Verification items for the finished model (mm, model axes). Coordinates: 2 decimals unless noted, no trailing zeros. Order: outer loops, then holes, each group sorted by start corner. A loop starts at its lowest first (then second) coordinate and runs counter-clockwise, first axis right, second up. Notation, with made-up numbers: (-40, 40) -> (-11, 40) arc R10 cw to (-11, 47) -> close; hole circle Ø4 at (39.25, 49). An arc over 180 degrees is marked (long way). Write each question's results on one line, items separated by ' | '. Start each with the question number.
(1) Cross-section at D-D on x = -12.5. Enter the section's corners in (y, z).
(2) Draft check along X on faces 1 (the cylindrical face through (-5.69, 9.84, 78.54)), 2 (the flat face through (-9, 44, 81)), 3 (the flat face through (-71.5, 46, 78)). Enter one of: +X half, -X half, draft (parallel to the pull), parting line (faces both ways), or undercut.
(3) Thickness scan on probe 1 along Y at (x, z) = (-37.5, 79.15); probe 2 along Y at (x, z) = (-12.5, 78.4); probe 3 along X at (y, z) = (70, 78.9). Record the ranges inside material, lowest first. Write a range as [from, to].
(4) Cross-section at B-B on y = 45. Enter the section's corners in (x, z), and give its area (3 significant figures).
(5) Cross-section at C-C on z = 80.1. Give the number of separate pieces and of enclosed holes in the cut face, and give its area (3 significant figures).
(6) Cross-section at A-A on x = -54. Enter the section's corners in (y, z).
```python
from build123d import *

# Parameters (mm, degrees)
SKETCH_1_W          = 69.5
SKETCH_1_H          = 100
SKETCH_1_R          = 1.5
EXTRUDE_1_DEPTH     = 5
SKETCH_5_R          = 1.6
SKETCH_5_R_2        = 27.5
CUT_EXTRUDE_1_DEPTH = 6
SKETCH_6_W          = 5
SKETCH_6_H          = 100
EXTRUDE_2_DEPTH     = 4.5
SKETCH_7_W          = 74
SKETCH_7_H          = 5
CUT_EXTRUDE_2_DEPTH = 7
SKETCH_8_W          = 74
SKETCH_8_H          = 5
CUT_EXTRUDE_3_DEPTH = 7


with BuildPart() as part:
    # Эскиз1 → Бобышка-Вытянуть1 (new body)
    with BuildSketch(Plane.XY.offset(81)):
        with Locations((-32.25, 45)):
            Rectangle(SKETCH_1_W, SKETCH_1_H)
        with Locations((-60, 8.5)):
            Circle(SKETCH_1_R, mode=Mode.SUBTRACT)
        with Locations((-60, 81.5)):
            Circle(SKETCH_1_R, mode=Mode.SUBTRACT)
        with Locations((-4.5, 79.25)):
            Circle(SKETCH_1_R, mode=Mode.SUBTRACT)
        with Locations((-4.5, 10.75)):
            Circle(SKETCH_1_R, mode=Mode.SUBTRACT)
    extrude(amount=-EXTRUDE_1_DEPTH)

    # Эскиз5 → Вырез-Вытянуть1 (cut, through all)
    with BuildSketch(Plane.XY.offset(81)):
        with Locations((-12.5, 70)):
            Circle(SKETCH_5_R)
        with Locations((-12.5, 20)):
            Circle(SKETCH_5_R)
        with Locations((-62.5, 20)):
            Circle(SKETCH_5_R)
        with Locations((-62.5, 70)):
            Circle(SKETCH_5_R)
        with Locations((-37.5, 45)):
            Circle(SKETCH_5_R_2)
    extrude(amount=-CUT_EXTRUDE_1_DEPTH, mode=Mode.SUBTRACT)

    # Эскиз6 → Бобышка-Вытянуть2 (add)
    with BuildSketch(Plane.ZY.offset(67)):
        with Locations((78.5, 45)):
            Rectangle(SKETCH_6_W, SKETCH_6_H)
    extrude(amount=EXTRUDE_2_DEPTH)

    # Эскиз7 → Вырез-Вытянуть2 (cut)
    with BuildSketch(Plane(origin=(0, 95, 0), x_dir=(1, 0, 0), z_dir=(0, 1, 0))):
        with Locations((-34.5, -78.5)):
            Rectangle(SKETCH_7_W, SKETCH_7_H)
    extrude(amount=-CUT_EXTRUDE_2_DEPTH, mode=Mode.SUBTRACT)

    # Эскиз8 → Вырез-Вытянуть3 (cut)
    with BuildSketch(Plane.XZ.offset(5)):
        with Locations((-34.5, 78.5)):
            Rectangle(SKETCH_8_W, SKETCH_8_H)
    extrude(amount=-CUT_EXTRUDE_3_DEPTH, mode=Mode.SUBTRACT)


solid = part.part
```
Results are:
1) outline: (2, 76) -> (18.4, 76) -> (18.4, 81) -> (2, 81) -> close; (21.6, 76) -> (33.54, 76) -> (33.54, 81) -> (21.6, 81) -> close; (56.46, 76) -> (68.4, 76) -> (68.4, 81) -> (56.46, 81) -> close; (71.6, 76) -> (88, 76) -> (88, 81) -> (71.6, 81) -> close
2) face 1: undercut | face 2: draft | face 3: -X half
3) probe 1: y = [2, 17.5], [72.5, 88] | probe 2: y = [2, 18.4], [21.6, 33.54], [56.46, 68.4], [71.6, 88] | probe 3: x = [-71.5, -64.1], [-60.9, -48.96], [-26.04, -14.1], [-10.9, 2.5]
4) outline: (-71.5, 76) -> (-65, 76) -> (-65, 81) -> (-71.5, 81) -> close; (-10, 76) -> (2.5, 76) -> (2.5, 81) -> (-10, 81) -> close | area: 95.0 mm2
5) separate pieces: 1 | enclosed holes: 9 | area: 3,930 mm2
6) outline: (2, 76) -> (23, 76) -> (23, 81) -> (2, 81) -> close; (67, 76) -> (88, 76) -> (88, 81) -> (67, 81) -> close
